The listing builds one solid part. Answer for the finished solid, in the listing's coordinates (mm). Give positions to 0.01 mm unless a question says otherwise; leave off trailing zeros. Order: outer loops, then holes, each group sorted by start corner. A loop starts at its lowest first (then second) coordinate and runs counter-clockwise, first axis right, second up.
```python
from build123d import *

# Parameters (mm, degrees)
BOSS_EXTRUDE1_DEPTH = 2
CHAMFER1_SIZE       = 10
CHAMFER2_SIZE       = 10


with BuildPart() as part:
    # Sketch1 → Boss-Extrude1 (new body)
    with BuildSketch(Plane.XY):
        Polygon((80, 24.434280886), (82, 26.434280886), (88, 26.434280886), (90, 24.434280886), (90, 20), (93, 20), (93, 15), (90, 15), (90, 0), (90, -15), (93, -15), (93, -20), (90, -20), (90, -40), (175, -40), (175, -20), (172, -20), (172, -15), (175, -15), (175, 0), (175, 15), (172, 15), (172, 20), (175, 20), (175, 80), (12, 80), (12, 77), (7, 77), (7, 80), (-5, 80), (-17, 80), (-17, 77), (-22, 77), (-22, 80), (-35, 80), (-35, 0), (-22, 0), (-22, 3), (-17, 3), (-17, 0), (-5, 0), (7, 0), (7, 3), (12, 3), (12, 0), (80, 0), align=None)
    extrude(amount=BOSS_EXTRUDE1_DEPTH)

    # Chamfer1
    chamfer1_edges = [part.edges().sort_by_distance(p)[0] for p in [
        (-35, 0, 1),
        (-35, 80, 1),
        (175, 80, 1),
        (175, -40, 1),
        (90, -40, 1),
    ]]
    chamfer(chamfer1_edges, length=CHAMFER1_SIZE)

    # Chamfer2
    chamfer2_edges = [part.edges().sort_by_distance(p)[0] for p in [
        (80, 0, 1),
    ]]
    chamfer(chamfer2_edges, length=CHAMFER2_SIZE)


solid = part.part
```
1) Find section B-B (x = -5.5). Write down the section's boundary in (y, z), then the cut area to 3 significant figures.
Geometry says:
outline: (0, 0) - (80, 0) - (80, 2) - (0, 2) - close
area: 160 mm2
2) Given P1, Ø1, axis at x = 91.5, z = 0.5, coming from the -Y side; P2, Ø1, axis at y = 79, z = 0.5, coming from the -X side; P3, Ø1, axis at y = 78.5, z = 1, coming from the +X side, each flat-ended and moving along its own axis, determine where each tip first touches the part or whether it passes through.
Geometry says:
P1: stops at y = -32
P2: stops at x = -26.5
P3: stops at x = 167
3) For a pull along X with two mould halves and no side action, classify faces 1 (the flat face through (95, -35, 1)), 2 (the flat face through (69, 34, 0)), 3 (the flat face through (75, 5, 1)) as +X half, -X half, draft (parallel to the pull), parting line (faces both ways), or undercut.
Geometry says:
face 1: -X half
face 2: draft
face 3: undercut
4) Straight lines are drawn through the part: probe 1 along X at (y, z) = (2.5, 0.8); probe 2 along X at (y, z) = (18.5, 0.9); probe 3 along X at (y, z) = (13.5, 1.2). For each, find the intervals that lie inside material, in ascending order.
Geometry says:
probe 1: x = -27.5 to -22, -17 to 7, 12 to 72.5, 90 to 175
probe 2: x = -35 to 80, 93 to 172
probe 3: x = -35 to 80, 90 to 175
5) Find section C-C (y = -18). Write down the section's boundary in (x, z).
Geometry says:
outline: (93, 0) - (172, 0) - (172, 2) - (93, 2) - close
6) Find section A-A (y = 7.5). Write down the section's boundary in (x, z).
Geometry says:
outline: (-32.5, 0) - (77.5, 0) - (77.5, 2) - (-32.5, 2) - close; (90, 0) - (175, 0) - (175, 2) - (90, 2) - close
